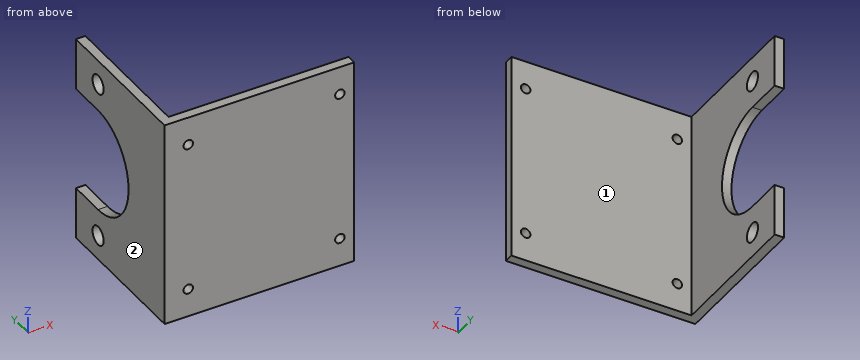
```python
from build123d import *

# Parameters (mm, degrees)
BOSS_EXTRUDE1_DEPTH = 69.85
CUT_EXTRUDE1_REACH  = 8.35
SKETCH2_R           = 6.35
CUT_EXTRUDE2_REACH  = 8.35
SKETCH3_R           = 3.175


with BuildPart() as part:
    # Sketch1 → Boss-Extrude1 (new body, symmetric)
    with BuildSketch(Plane.XY):
        Polygon((0, 0), (0, 95.25), (-6.35, 95.25), (-6.35, -6.35), (120.65, -6.35), (120.65, 0), align=None)
    extrude(amount=BOSS_EXTRUDE1_DEPTH, both=True)

    # Sketch2 → Cut-Extrude1 (cut, up to next)
    with BuildSketch(Plane(origin=(0, 0, 0), x_dir=(0, 0, -1), z_dir=(1, 0, 0)), mode=Mode.PRIVATE) as cut_extrude1_sk1:
        with Locations((-53.1876, 69.85)):
            Circle(SKETCH2_R)
    cut_extrude1_tool1 = extrude(cut_extrude1_sk1.sketch, amount=-CUT_EXTRUDE1_REACH, mode=Mode.PRIVATE) & part.part
    add(cut_extrude1_tool1.solids().sort_by_distance((0, 69.85, 53.1876))[0], mode=Mode.SUBTRACT)
    # Sketch2 → Cut-Extrude1 (cut, up to next)
    with BuildSketch(Plane(origin=(0, 0, 0), x_dir=(0, 0, -1), z_dir=(1, 0, 0)), mode=Mode.PRIVATE) as cut_extrude1_sk2:
        with Locations((53.1876, 69.85)):
            Circle(SKETCH2_R)
    cut_extrude1_tool2 = extrude(cut_extrude1_sk2.sketch, amount=-CUT_EXTRUDE1_REACH, mode=Mode.PRIVATE) & part.part
    add(cut_extrude1_tool2.solids().sort_by_distance((0, 69.85, -53.1876))[0], mode=Mode.SUBTRACT)
    # Sketch2 → Cut-Extrude1 (cut, up to next)
    with BuildSketch(Plane(origin=(0, 0, 0), x_dir=(0, 0, -1), z_dir=(1, 0, 0)), mode=Mode.PRIVATE) as cut_extrude1_sk3:
        with BuildLine():
            Line((-34.925, 69.85), (-34.925, 95.25))
            Line((-34.925, 95.25), (34.925, 95.25))
            Line((34.925, 95.25), (34.925, 69.85))
            ThreePointArc((34.925, 69.85), (0, 34.925), (-34.925, 69.85))
        make_face()
    cut_extrude1_tool3 = extrude(cut_extrude1_sk3.sketch, amount=-CUT_EXTRUDE1_REACH, mode=Mode.PRIVATE) & part.part
    add(cut_extrude1_tool3.solids().sort_by_distance((0, 68.259897, 0))[0], mode=Mode.SUBTRACT)

    # Sketch3 → Cut-Extrude2 (cut, up to next)
    with BuildSketch(Plane(origin=(0, 0, 0), x_dir=(1, 0, 0), z_dir=(0, 1, 0)), mode=Mode.PRIVATE) as cut_extrude2_sk1:
        with Locations((9.525, 50.8)):
            Circle(SKETCH3_R)
    cut_extrude2_tool1 = extrude(cut_extrude2_sk1.sketch, amount=-CUT_EXTRUDE2_REACH, mode=Mode.PRIVATE) & part.part
    add(cut_extrude2_tool1.solids().sort_by_distance((9.525, 0, -50.8))[0], mode=Mode.SUBTRACT)
    # Sketch3 → Cut-Extrude2 (cut, up to next)
    with BuildSketch(Plane(origin=(0, 0, 0), x_dir=(1, 0, 0), z_dir=(0, 1, 0)), mode=Mode.PRIVATE) as cut_extrude2_sk2:
        with Locations((111.125, 50.8)):
            Circle(SKETCH3_R)
    cut_extrude2_tool2 = extrude(cut_extrude2_sk2.sketch, amount=-CUT_EXTRUDE2_REACH, mode=Mode.PRIVATE) & part.part
    add(cut_extrude2_tool2.solids().sort_by_distance((111.125, 0, -50.8))[0], mode=Mode.SUBTRACT)
    # Sketch3 → Cut-Extrude2 (cut, up to next)
    with BuildSketch(Plane(origin=(0, 0, 0), x_dir=(1, 0, 0), z_dir=(0, 1, 0)), mode=Mode.PRIVATE) as cut_extrude2_sk3:
        with Locations((9.525, -50.8)):
            Circle(SKETCH3_R)
    cut_extrude2_tool3 = extrude(cut_extrude2_sk3.sketch, amount=-CUT_EXTRUDE2_REACH, mode=Mode.PRIVATE) & part.part
    add(cut_extrude2_tool3.solids().sort_by_distance((9.525, 0, 50.8))[0], mode=Mode.SUBTRACT)
    # Sketch3 → Cut-Extrude2 (cut, up to next)
    with BuildSketch(Plane(origin=(0, 0, 0), x_dir=(1, 0, 0), z_dir=(0, 1, 0)), mode=Mode.PRIVATE) as cut_extrude2_sk4:
        with Locations((111.125, -50.8)):
            Circle(SKETCH3_R)
    cut_extrude2_tool4 = extrude(cut_extrude2_sk4.sketch, amount=-CUT_EXTRUDE2_REACH, mode=Mode.PRIVATE) & part.part
    add(cut_extrude2_tool4.solids().sort_by_distance((111.125, 0, 50.8))[0], mode=Mode.SUBTRACT)


solid = part.part
```
Design review of the part built by this model. Coordinates are the model's own, in mm. Face numbers are marked on the shaded views. A direction names the side the tool comes from. Give positions to 0.01 mm unless a question says otherwise; leave off trailing zeros. Write each loop counter-clockwise with the first axis right and the second up, starting at its lowest first coordinate (ties: lowest second). Pieces come first, ordered by that corner, then holes. Notation, with made-up numbers: (-3.75, 79) -> (10.25, 79) arc R11 ccw to (10.25, 96) -> close; hole circle Ø4 at (-24.5, -30.75). An arc over 180 degrees is marked (long way). Answer in a Markdown table with one row per item.
(1) To check wall thickness, follow probe 1 along X at (y, z) = (-3.5, 50.8); probe 2 along Z at (x, y) = (7.5, -1); probe 3 along Z at (x, y) = (-3, 69). State the ranges of each line that lie inside material, in increasing order.
Results:
| item | result |
|---|---|
| probe 1 | -6.35 to 6.35, 12.7 to 107.95, 114.3 to 120.65 |
| probe 2 | -69.85 to -53.25, -48.35 to 48.35, 53.25 to 69.85 |
| probe 3 | -69.85 to -59.48, -46.89 to -34.91, 34.91 to 46.89, 59.48 to 69.85 |
(2) For the marked faces 1 and 2, list the 3-axis set-ups (+Z, -Z, +X, -X, +Y, -Y) from which the entire face can be reached by the end or side of a thin tool; tool diameter is ignored.
Results:
| item | result |
|---|---|
| face 1 | +Z, -Z, +X, +Y |
| face 2 | +Z, -Z, -X, +Y, -Y |
(3) Consider section B-B (y = 41). State the section outline as (x, z) points.
Results:
| item | result |
|---|---|
| outline | (-6.35, -69.85) -> (0, -69.85) -> (0, -19.68) -> (-6.35, -19.68) -> close; (-6.35, 19.68) -> (0, 19.68) -> (0, 69.85) -> (-6.35, 69.85) -> close |
(4) Clearance check with flat-ended pins moving along their axes: pin 1 (8.5 mm diameter, centred on x = 9.525, z = -50.8, fed in from +Y); pin 2 (12 mm diameter, centred on y = 33, z = -13, fed in from +X); pin 3 (8.5 mm diameter, centred on x = 9.525, z = 50.8, fed in from -Y). State where each tip first meets the part, or that it passes through.
Results:
| item | result |
|---|---|
| pin 1 | y = 0 |
| pin 2 | x = 0 |
| pin 3 | y = -6.35 |
(5) Consider section C-C (y = 73). State the section outline as (x, z) points (3 decimals), then the cut area to 3 significant figures.
Results:
| item | result |
|---|---|
| outline | (-6.35, -69.85) -> (0, -69.85) -> (0, -58.701) -> (-6.35, -58.701) -> close; (-6.35, -47.674) -> (0, -47.674) -> (0, -34.925) -> (-6.35, -34.925) -> close; (-6.35, 34.925) -> (0, 34.925) -> (0, 47.674) -> (-6.35, 47.674) -> close; (-6.35, 58.701) -> (0, 58.701) -> (0, 69.85) -> (-6.35, 69.85) -> close |
| area | 304 mm2 |
(6) Consider section A-A (z = -50.8). State the section outline as (x, y) points, then the cut area to 3 significant figures.
Results:
| item | result |
|---|---|
| outline | (-6.35, -6.35) -> (6.35, -6.35) -> (6.35, 0) -> (0, 0) -> (0, 63.97) -> (-6.35, 63.97) -> close; (-6.35, 75.73) -> (0, 75.73) -> (0, 95.25) -> (-6.35, 95.25) -> close; (12.7, -6.35) -> (107.95, -6.35) -> (107.95, 0) -> (12.7, 0) -> close; (114.3, -6.35) -> (120.65, -6.35) -> (120.65, 0) -> (114.3, 0) -> close |
| area | 1,260 mm2 |
(7) Consider section D-D (z = 0). State the section outline as (x, y) points (3 decimals), then the cut area to 3 significant figures.
Results:
| item | result |
|---|---|
| outline | (-6.35, -6.35) -> (120.65, -6.35) -> (120.65, 0) -> (0, 0) -> (0, 34.925) -> (-6.35, 34.925) -> close |
| area | 1,030 mm2 |
